Verification items for the finished model (mm, model axes). Coordinates: 2 decimals unless noted, no trailing zeros.
Q1. Mould release check, pull along Y, two halves, no side actions. Record for faces 1 (the face through (0, 38, 0)), 2 (the face through (-61.56, 10.07, 0.76)): +Y half, -Y half, draft (parallel to the pull), parting line (faces both ways), or undercut.
Q2. Material ranges on probe 1 along X at (y, z) = (64.5, 0.35), recorded low to high.
Q3. Go/stop test with flat-tipped pins: P1, Ø4, axis at x = -43.46, y = 18, coming from the +Z side; P2, Ø3, axis at x = 66.54, y = 12, coming from the -Z side. Record where each tip stops, or that it passes through.
```python
from build123d import *

# Parameters (mm, degrees)
SKETCH1_W           = 141.5
SKETCH1_H           = 74.5
BOSS_EXTRUDE1_DEPTH = 1.5
SKETCH2_R           = 1.6
CUT_EXTRUDE1_DEPTH  = 1.5
SKETCH3_R           = 1.6
CUT_EXTRUDE2_DEPTH  = 1.5
SKETCH4_R           = 1.6
CUT_EXTRUDE3_DEPTH  = 1.5


with BuildPart() as part:
    # Sketch1 → Boss-Extrude1 (new body)
    with BuildSketch(Plane.XY):
        with Locations((0.787232686, 37.25)):
            Rectangle(SKETCH1_W, SKETCH1_H)
    extrude(amount=BOSS_EXTRUDE1_DEPTH)

    # Sketch2 → Cut-Extrude1 (cut)
    with BuildSketch(Plane.XY.offset(1.5)):
        with Locations((-59.962767314, 64.5)):
            Circle(SKETCH2_R)
        with Locations((-59.962767314, 10)):
            Circle(SKETCH2_R)
    extrude(amount=-CUT_EXTRUDE1_DEPTH, mode=Mode.SUBTRACT)

    # Sketch3 → Cut-Extrude2 (cut)
    with BuildSketch(Plane.XY.offset(1.5)):
        with Locations((66.537232686, 62.5)):
            Circle(SKETCH3_R)
        with Locations((66.537232686, 12)):
            Circle(SKETCH3_R)
    extrude(amount=-CUT_EXTRUDE2_DEPTH, mode=Mode.SUBTRACT)

    # Sketch4 → Cut-Extrude3 (cut)
    with BuildSketch(Plane.XY.offset(1.5)):
        with Locations((-43.462767314, 18)):
            Circle(SKETCH4_R)
    extrude(amount=-CUT_EXTRUDE3_DEPTH, mode=Mode.SUBTRACT)


solid = part.part
```
Geometry check:
1. face 1: draft
1. face 2: undercut
2. probe 1: x = -69.96 to -61.56, -58.36 to 71.54
3. P1: stops at z = 1.5
3. P2: passes through
